Input: part model. Units: mm. Frame: model coordinates. Coordinates: 2 decimals unless noted, no trailing zeros. Loops run counter-clockwise (first coordinate to the right, second up) from the corner with the lowest first, then second, coordinate; pieces in that order, holes last.
Item 1: Ray query, line 1 along Z through (x, y) = (0, 1.7); line 2 along Z through (x, y) = (0.5, 1.3); line 3 along X through (y, z) = (1.25, 0). Return the intervals inside material, ascending.
Item 2: Section D-D on z = -4. Return loops of the section in (x, y).
Item 3: Section C-C on x = 0. Return loops of the section in (y, z), and give its area (3 significant figures).
Item 4: Section A-A on y = 2.7. Return loops of the section in (x, z) (3 decimals), and give its area (3 significant figures).
Item 5: Section B-B on z = -70. Return loops of the section in (x, y).
Item 6: Contact query for flat-ended pins moving along their axis: P1, Ø2, axis at x = -2, y = 3.5, coming from the +Z side; P2, Ø1, axis at y = 2, z = -92, coming from the +X side; P3, Ø1, axis at y = 3.5, z = -48.5, coming from the +X side. Output: stop coordinate, or through.
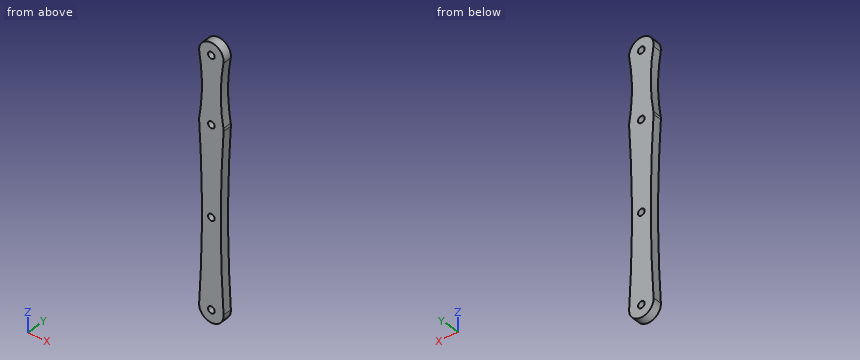
```python
from build123d import *

# Parameters (mm, degrees)
SKETCH1_R           = 1.5
BOSS_EXTRUDE1_DEPTH = 4


with BuildPart() as part:
    # Sketch1 → Boss-Extrude1 (new body)
    with BuildSketch(Plane(origin=(0, 0, 0), x_dir=(1, 0, 0), z_dir=(0, 1, 0))):
        with BuildLine():
            ThreePointArc((-5.424137931, 0.910344828), (0, -5.5), (5.424137931, 0.910344828))
            ThreePointArc((5.424137931, 0.910344828), (4.25, 15), (5.424137931, 29.089655172))
            ThreePointArc((5.424137931, 29.089655172), (5.492593836, 29.71467045), (5.489268293, 30.343414634))
            ThreePointArc((5.489268293, 30.343414634), (4.25, 70), (5.489268293, 109.656585366))
            ThreePointArc((5.489268293, 109.656585366), (0, 115.5), (-5.489268293, 109.656585366))
            ThreePointArc((-5.489268293, 109.656585366), (-4.25, 70), (-5.489268293, 30.343414634))
            ThreePointArc((-5.489268293, 30.343414634), (-5.492593836, 29.71467045), (-5.424137931, 29.089655172))
            ThreePointArc((-5.424137931, 29.089655172), (-4.25, 15), (-5.424137931, 0.910344828))
        make_face()
        Circle(SKETCH1_R, mode=Mode.SUBTRACT)
        with Locations((0, 110)):
            Circle(SKETCH1_R, mode=Mode.SUBTRACT)
        with Locations((0, 30)):
            Circle(SKETCH1_R, mode=Mode.SUBTRACT)
        with Locations((0, 70)):
            Circle(SKETCH1_R, mode=Mode.SUBTRACT)
    extrude(amount=BOSS_EXTRUDE1_DEPTH)


solid = part.part
```
Results found:
1. line 1: z = -115.5 to -111.5, -108.5 to -71.5, -68.5 to -31.5, -28.5 to -1.5, 1.5 to 5.5
1. line 2: z = -115.48 to -111.41, -108.59 to -71.41, -68.59 to -31.41, -28.59 to -1.41, 1.41 to 5.48
1. line 3: x = -5.5 to -1.5, 1.5 to 5.5
2. outline: (-4.96, 0) - (4.96, 0) - (4.96, 4) - (-4.96, 4) - close
3. outline: (0, -115.5) - (4, -115.5) - (4, -111.5) - (0, -111.5) - close; (0, -108.5) - (4, -108.5) - (4, -71.5) - (0, -71.5) - close; (0, -68.5) - (4, -68.5) - (4, -31.5) - (0, -31.5) - close; (0, -28.5) - (4, -28.5) - (4, -1.5) - (0, -1.5) - close; (0, 1.5) - (4, 1.5) - (4, 5.5) - (0, 5.5) - close
3. area: 436 mm2
4. outline: (-5.489, -109.657) arc R5.5 ccw (long way) to (5.489, -109.657) arc R635.125 cw to (5.489, -30.343) arc R5.5 ccw to (5.424, -29.09) arc R85.125 cw to (5.424, -0.91) arc R5.5 ccw (long way) to (-5.424, -0.91) arc R85.125 cw to (-5.424, -29.09) arc R5.5 ccw to (-5.489, -30.343) arc R635.125 cw to start; hole circle Ø3 at (0, -110); hole circle Ø3 at (0, -70); hole circle Ø3 at (0, -30); hole circle Ø3 at (0, 0)
4. area: 1,100 mm2
5. outline: (-4.25, 0) - (-1.5, 0) - (-1.5, 4) - (-4.25, 4) - close; (1.5, 0) - (4.25, 0) - (4.25, 4) - (1.5, 4) - close
6. P1: stops at z = 5.41
6. P2: stops at x = 4.65
6. P3: stops at x = 4.63
